Part print with two shaded views. Sizes in mm from the minimum x, y, z corner. A direction names the side the tool comes from. Coordinates: 2 decimals unless noted, no trailing zeros. Write each loop counter-clockwise with the first axis right and the second up, starting at its lowest first coordinate (ties: lowest second). Pieces come first, ordered by that corner, then holes. Notation, with made-up numbers: (9.5, 68.25) -> (16.5, 68.25) arc R30 cw to (16.5, 91.25) -> close; hole circle Ø10 at (-37, 62.25). An arc over 180 degrees is marked (long way). Write item = value, one per line. Start each with the question number.
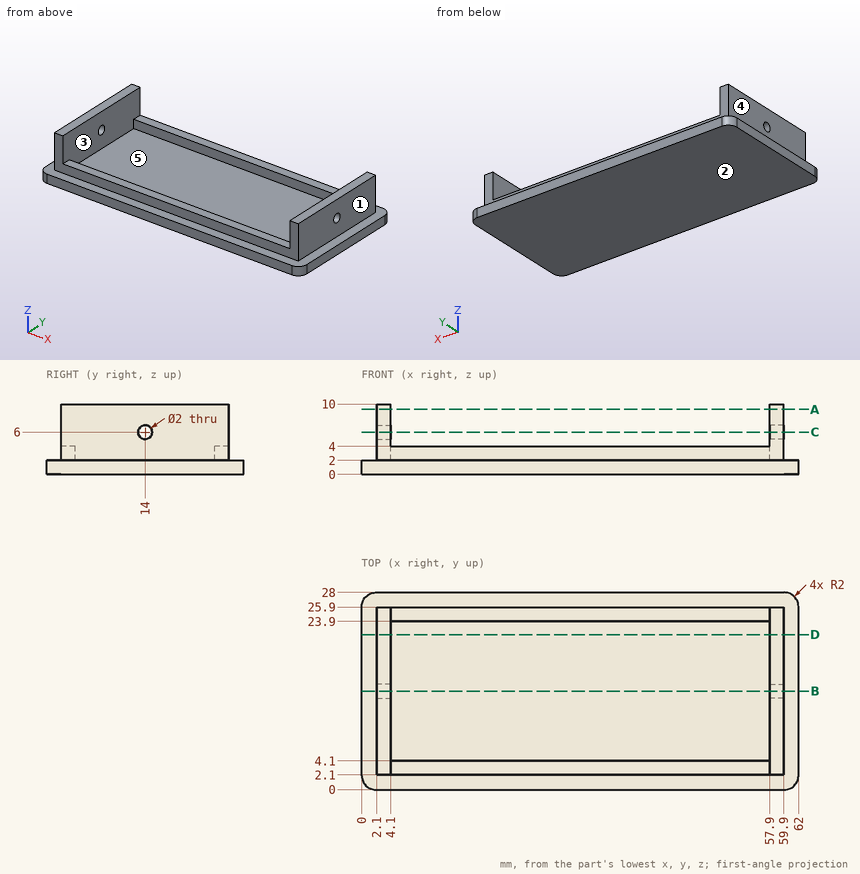
(1) 3-axis set-ups, long thin cutter, end or side, ignore diameter. For the marked faces 1, 2 and 3: which of +Z, -Z, +X, -X, +Y, -Y reach the whole face in a straight line?
(2) Saw through at B-B (y = 14). Give the cut face in (x, z).
(3) Drop flat-ended pins along their axis: pin 1 Ø3 at (y, z) = (14, 6) entering from +X; pin 2 Ø1.6 at (x, y) = (37.5, 2.5) entering from +Z; pin 3 Ø5 at (x, y) = (46.5, 15) entering from -Z; pin 4 Ø0.6 at (x, z) = (21.5, 3) entering from -Y. Give the stop position or say it passes through.
(4) Saw through at A-A (z = 9.25). Give the cut face in (x, y).
(5) Saw through at D-D (y = 22). Give the cut face in (x, z), then the cut area to 3 significant figures.
(6) Saw through at C-C (z = 6). Give the cut face in (x, y).
(7) Mould opens along Y. For the marked faces 4 and 5 say: released by +Y, released by -Y, zero draft, split by the parting line, or undercut.
(8) Drill centre lines: line 1 along X through (y, z) = (3.5, 9.5); line 2 along Y through (x, z) = (58.95, 6); line 3 along Z through (x, y) = (59.05, 14). Where is each one in solid material? Low to high.
Returned:
q1.face_1 = +Z, +X, +Y, -Y
q1.face_2 = -Z, +X, -X, +Y, -Y
q1.face_3 = +Z
q2.outline = (0, 0) -> (62, 0) -> (62, 2) -> (59.9, 2) -> (59.9, 5) -> (57.9, 5) -> (57.9, 2) -> (4.1, 2) -> (4.1, 5) -> (2.1, 5) -> (2.1, 2) -> (0, 2) -> close; (2.1, 7) -> (4.1, 7) -> (4.1, 10) -> (2.1, 10) -> close; (57.9, 7) -> (59.9, 7) -> (59.9, 10) -> (57.9, 10) -> close
q3.pin_1 = 59.9
q3.pin_2 = 4
q3.pin_3 = 0
q3.pin_4 = 2.1
q4.outline = (2.1, 2.1) -> (4.1, 2.1) -> (4.1, 25.9) -> (2.1, 25.9) -> close; (57.9, 2.1) -> (59.9, 2.1) -> (59.9, 25.9) -> (57.9, 25.9) -> close
q5.outline = (0, 0) -> (62, 0) -> (62, 2) -> (59.9, 2) -> (59.9, 10) -> (57.9, 10) -> (57.9, 2) -> (4.1, 2) -> (4.1, 10) -> (2.1, 10) -> (2.1, 2) -> (0, 2) -> close
q5.area = 156 mm2
q6.outline = (2.1, 2.1) -> (4.1, 2.1) -> (4.1, 13) -> (2.1, 13) -> close; (2.1, 15) -> (4.1, 15) -> (4.1, 25.9) -> (2.1, 25.9) -> close; (57.9, 2.1) -> (59.9, 2.1) -> (59.9, 13) -> (57.9, 13) -> close; (57.9, 15) -> (59.9, 15) -> (59.9, 25.9) -> (57.9, 25.9) -> close
q7.face_4 = zero draft
q7.face_5 = undercut
q8.line_1 = 2.1 to 4.1, 57.9 to 59.9
q8.line_2 = 2.1 to 13, 15 to 25.9
q8.line_3 = 0 to 5, 7 to 10
